Could you check a few things on this drawing? It's one solid part, dimensions in mm from its lowest x, y, z. Give positions to 0.01 mm unless a question says otherwise; leave off trailing zeros. Loops run counter-clockwise (first coordinate to the right, second up) from the corner with the lowest first, then second, coordinate; pieces in that order, holes last. Notation, with made-up numbers: (78, 86) - (133, 86) arc R24 ccw to (133, 101) - close; hole circle Ø9 at (73.5, 38). An arc over 180 degrees is marked (long way). Write item = value, one per line.
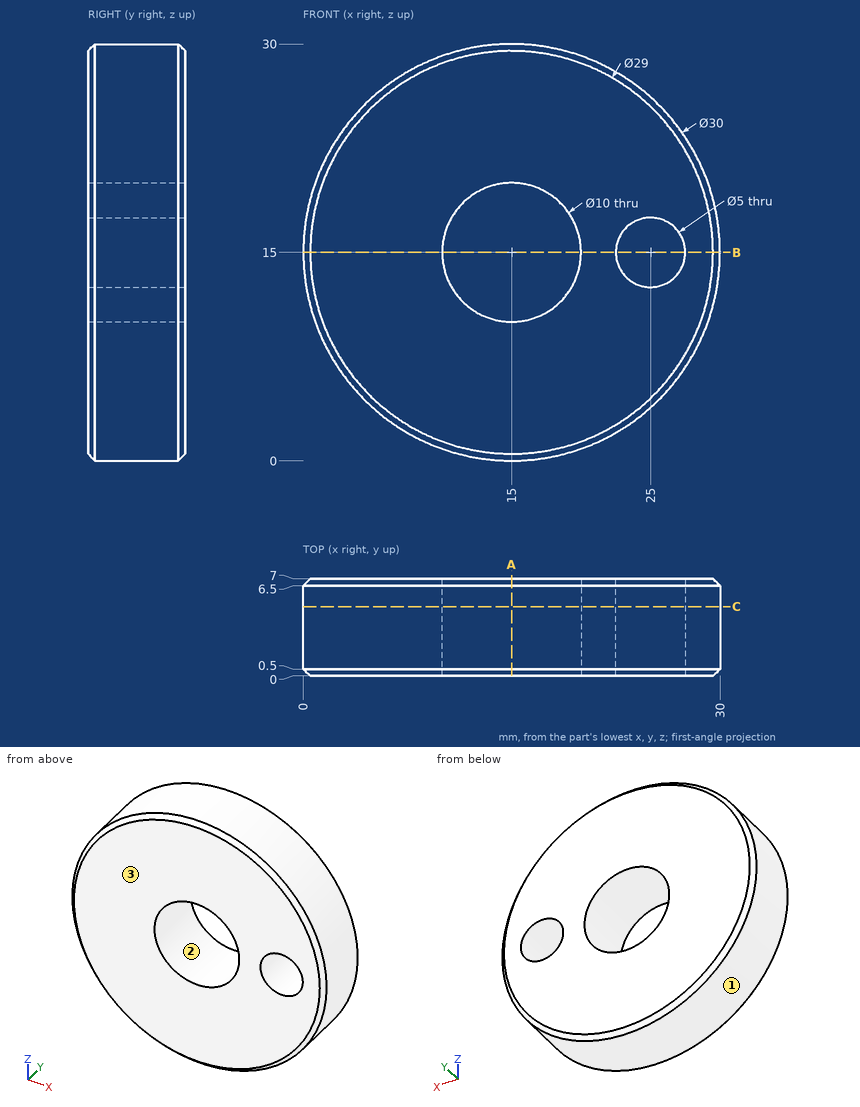
Q1. Imagine slicing it at A-A, the plane x = 15. Write out the boundary of the cut face in (y, z).
Output:
outline = (0, 0.5) - (0.5, 0) - (6.5, 0) - (7, 0.5) - (7, 10) - (0, 10) - close; (0, 20) - (7, 20) - (7, 29.5) - (6.5, 30) - (0.5, 30) - (0, 29.5) - close
Q2. Imagine slicing it at C-C, the plane y = 5. Write out the boundary of the cut face in (x, z).
Output:
outline = circle Ø30 at (15, 15); hole circle Ø10 at (15, 15); hole circle Ø5 at (25, 15)
Q3. I need wall thicknesses on L1, parallel to Z at x = 15, y = 4; L2, parallel to Z at x = 25, y = 3; L3, parallel to Z at x = 22.25, y = 1.25. Which ranges of each line are inside material? Lowest first, please.
Output:
L1 = 0 to 10, 20 to 30
L2 = 3.82 to 12.5, 17.5 to 26.18
L3 = 1.87 to 28.13
Q4. We'd pull the mould along Z, two halves only. Please class the marked faces 1, 2 and 3: released by +Z, released by -Z, zero draft, split by the parting line, or undercut.
Output:
face_1 = split by the parting line
face_2 = undercut
face_3 = zero draft
Q5. For pin 1 (6 mm diameter, centred on x = 15, z = 15, fed in from +Y); pin 2 (2 mm diameter, centred on x = 9.5, y = 6, fed in from +Z); pin 3 (1 mm diameter, centred on y = 6, z = 10, fed in from -X), each with a flat end and sliding along its axis, tell me the tip position at first contact or that it passes through.
Output:
pin_1 = through
pin_2 = 29.31
pin_3 = 0.69
Q6. Imagine slicing it at B-B, the plane z = 15. Write out the boundary of the cut face in (x, y), then the cut area to 4 significant figures.
Output:
outline = (0, 0.5) - (0.5, 0) - (10, 0) - (10, 7) - (0.5, 7) - (0, 6.5) - close; (20, 0) - (22.5, 0) - (22.5, 7) - (20, 7) - close; (27.5, 0) - (29.5, 0) - (30, 0.5) - (30, 6.5) - (29.5, 7) - (27.5, 7) - close
area = 104.5 mm2
